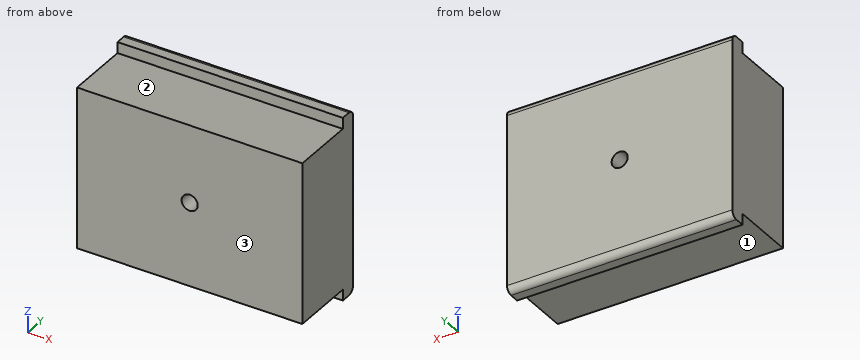
```python
from build123d import *

# Parameters (mm, degrees)
BOSS_EXTRUDE1_DEPTH = 1778
SKETCH2_R           = 63.5
CUT_EXTRUDE1_DEPTH  = 1778


with BuildPart() as part:
    # Sketch1 → Boss-Extrude1 (new body)
    with BuildSketch(Plane(origin=(0, 0, 0), x_dir=(0, 0, -1), z_dir=(1, 0, 0))):
        with BuildLine():
            Line((0, 0), (1270, 0))
            Line((1270, 0), (1270, 508))
            Line((1270, 508), (1357.172672295, 508))
            Line((1357.172672295, 508), (1357.172672295, 584.2))
            ThreePointArc((1357.172672295, 584.2), (1342.293696779, 620.121024484), (1306.372672295, 635))
            Line((1306.372672295, 635), (-36.372672295, 635))
            ThreePointArc((-36.372672295, 635), (-72.293696779, 620.121024484), (-87.172672295, 584.2))
            Line((-87.172672295, 584.2), (-87.172672295, 508))
            Line((-87.172672295, 508), (0, 508))
            Line((0, 508), (0, 0))
        make_face()
    extrude(amount=BOSS_EXTRUDE1_DEPTH)

    # Sketch2 → Cut-Extrude1 (cut)
    with BuildSketch(Plane(origin=(0, 635, 0), x_dir=(1, 0, 0), z_dir=(0, 1, 0))):
        with Locations(Location((889, 611.327327705, 0), (0, 0, 270))):
            Circle(SKETCH2_R)
    extrude(amount=-CUT_EXTRUDE1_DEPTH, mode=Mode.SUBTRACT)


solid = part.part
```
Part model, mm, in its own coordinate system. Face numbers are marked on the shaded views. A direction names the side the tool comes from. Round coordinates to 2 decimals unless told otherwise and drop trailing zeros. Write each loop counter-clockwise with the first axis right and the second up, starting at its lowest first coordinate (ties: lowest second). Pieces come first, ordered by that corner, then holes. Notation, with made-up numbers: (3, 6.5) -> (51, 6.5) arc R26 ccw to (51, 20.5) -> close; hole circle Ø11 at (45, 54.25). An arc over 180 degrees is marked (long way). Return JSON: item names as keys, results as strings. Group by question number.
Q1. Which spindle directions (+Z, -Z, +X, -X, +Y, -Y) get a long thin tool onto all of the face, cutting with end or side? Do the marked faces 1, 2 and 3. Say none if no direction does.
Q2. Saw through at B-B on y = 383.5. Write the cut outline in (x, z), plus the area to 3 significant figures.
Q3. Probe L1, parallel to Z at x = 1128.5, y = 478; L2, parallel to X at y = 371, z = -574; L3, parallel to X at y = 379, z = -639.5. List the from-to ranges inside material, lowest first. Write a range as [from, to].
Q4. Saw through at A-A on x = 889. Write the cut outline in (y, z), plus the area to 3 significant figures.
Q5. Pin check, flat tips, straight feed: pin 1 (1 mm diameter, centred on x = 204.5, y = 258, fed in from -Z); pin 2 (1 mm diameter, centred on x = 556.5, y = 169.5, fed in from +Z). Stop position of each tip, or through.
Answer:
{
 "1": {"face 1": "-Z, +X, -X, -Y", "face 2": "+Z, +X, -X, -Y", "face 3": "+Z, -Z, +X, -X, -Y"},
 "2": {"outline": "(0, -1270) -> (1778, -1270) -> (1778, 0) -> (0, 0) -> close; hole circle Ø127 at (889, -611.33)", "area": "2,250,000 mm2"},
 "3": {"L1": "[-1270, 0]", "L2": "[0, 837.63], [940.37, 1778]", "L3": "[0, 832.09], [945.91, 1778]"},
 "4": {"outline": "(0, -1270) -> (508, -1270) -> (508, -1357.17) -> (584.2, -1357.17) arc R50.8 ccw to (635, -1306.37) -> (635, -674.83) -> (0, -674.83) -> close; (0, -547.83) -> (635, -547.83) -> (635, 36.37) arc R50.8 ccw to (584.2, 87.17) -> (508, 87.17) -> (508, 0) -> (0, 0) -> close", "area": "747,000 mm2"},
 "5": {"pin 1": "z = -1270", "pin 2": "z = 0"}
}
